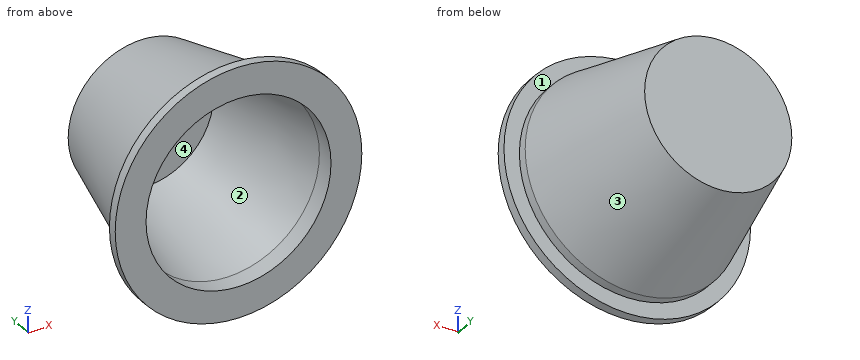
```python
from build123d import *

# Parameters (mm, degrees)
F0_R     = 40
F0_R_2   = 30
F1_DEPTH = 3
F2_R     = 35
F2_R_2   = 30
F3_DEPTH = 3
F5_R     = 23.875
F6_R     = 35
F9_R     = 22
F10_R    = 30


with BuildPart() as f1:
    # F0 (on Front) → F1 (new body)
    with BuildSketch(Plane.XZ):
        Circle(F0_R)
        Circle(F0_R_2, mode=Mode.SUBTRACT)
    extrude(amount=F1_DEPTH)

    # F2 (on Front) → F3 (join)
    with BuildSketch(Plane.XZ):
        Circle(F2_R)
        Circle(F2_R_2, mode=Mode.SUBTRACT)
    extrude(amount=-F3_DEPTH)

    # F5 (on offset) → F7 section 0
    with BuildSketch(Plane.XZ.offset(-47.05)):
        Circle(F5_R)
    # F6 (on face) → F7 section 1
    with BuildSketch(Plane(origin=(0, 3, 0), x_dir=(-1, 0, 0), z_dir=(0, 1, 0))):
        Circle(F6_R)
    loft()

    # F9 (on offset) → F11 section 0
    with BuildSketch(Plane.XZ.offset(-45)):
        Circle(F9_R)
    # F10 (on face) → F11 section 1
    with BuildSketch(Plane.XZ.offset(-3)):
        Circle(F10_R)
    loft(mode=Mode.SUBTRACT)


solid = f1.part
```
Geometry check sheet. Reference: the model listing, model coordinates, mm. Face numbers are marked on the shaded views. Round coordinates to 2 decimals unless told otherwise and drop trailing zeros. Order: outer loops, then holes, each group sorted by start corner. A loop starts at its lowest first (then second) coordinate and runs counter-clockwise, first axis right, second up. Notation, with made-up numbers: (10, -15) -> (19, -15) arc R30 ccw to (19, 19) -> close; hole circle Ø5 at (51.5, 0). An arc over 180 degrees is marked (long way). Return JSON: item names as keys, results as strings. Group by question number.
Q1. Section check C-C, the plane y = 6. Record the boundary of the cut face in (x, z).
Q2. Material ranges on probe 1 along Z at (x, y) = (0, -0.3); probe 2 along Z at (x, y) = (0, 1.55); probe 3 along Y at (x, z) = (-5.5, -14), recorded low to high. Write a range as from..to.
Q3. Release check for a two-part mould opening along Z. For the marked faces 1, 2, 3 and 4 record: released by +Z, released by -Z, zero draft, split by the parting line, or undercut.
Q4. Section check A-A, the plane x = 0. Record the boundary of the cut face in (y, z) (3 decimals), plus the area to 3 significant figures.
Q5. Gauge pin test, flat ends, axial feed: pin 1 (2 mm diameter, centred on y = 15, z = 20.5, fed in from +X); pin 2 (8 mm diameter, centred on x = -4.5, z = 15.5, fed in from -Y); pin 3 (4 mm diameter, centred on x = -10, y = 9, fed in from +Z). Record the tip position at first contact, or that the pin passes through.
Q6. Section check B-B, the plane y = 34.5. Record the boundary of the cut face in (x, z).
Numbers:
{
 "1": {"outline": "circle Ø68.48 at (0, 0); hole circle Ø58.86 at (0, 0)"},
 "2": {"probe 1": "-40..-30, 30..40", "probe 2": "-35..-30, 30..35", "probe 3": "45..47.05"},
 "3": {"face 1": "zero draft", "face 2": "undercut", "face 3": "split by the parting line", "face 4": "undercut"},
 "4": {"outline": "(-3, -40) -> (0, -40) -> (0, -35) -> (3, -35) -> (47.05, -23.875) -> (47.05, 23.875) -> (3, 35) -> (0, 35) -> (0, 40) -> (-3, 40) -> (-3, 30) -> (3, 30) -> (45, 22) -> (45, -22) -> (3, -30) -> (-3, -30) -> close", "area": "499 mm^2"},
 "5": {"pin 1": "x = 25.4", "pin 2": "y = 45", "pin 3": "z = 32.73"},
 "6": {"outline": "circle Ø54.09 at (0, 0); hole circle Ø48 at (0, 0)"}
}
